Design review of the part shown in the three views and the two pictorial views. Dimensions are in mm from the part's minimum x, y and z. A direction names the side the tool comes from. Give positions to 0.01 mm unless a question says otherwise; leave off trailing zeros. Order: outer loops, then holes, each group sorted by start corner. A loop starts at its lowest first (then second) coordinate and runs counter-clockwise, first axis right, second up.
Item 1: Consider section B-B (y = 12). Give the boundary of the cut face in (x, z), plus the area to 3 significant figures.
Item 2: The part is to be moulded in two halves that separate along X. For the marked faces 1, 2 and 3, say which applies: released by +X, released by -X, zero draft, split by the parting line, or undercut.
Item 3: For probe 1 along Y at (x, z) = (12, 4.4); probe 2 along Z at (x, y) = (12, 14.5); probe 3 along X at (y, z) = (12.25, 9), list the stretches that pass through material, from the lowest coordinate up.
Item 4: Consider section A-A (x = 12). Give the boundary of the cut face in (y, z), plus the area to 3 significant figures.
Item 5: Consider section C-C (z = 7). Give the boundary of the cut face in (x, y).
Item 6: For P1, Ø1.5, axis at x = 5.5, y = 15, coming from the -Z side (1 decimal); P2, Ø8, axis at x = 15.5, y = 6, coming from the -Z side; P3, Ø1, axis at x = 5, z = 10.5, coming from the +Y side; P4, Ø2, axis at x = 3.5, y = 17, coming from the +Z side, all flat-tipped, find the tip position at first contact; note any pin that passes through.
Item 7: Consider section D-D (x = 18.75). Give the boundary of the cut face in (y, z).
Item 8: Machinability: for the marked faces 4 and 5, which of the approach directions +Z, -Z, +X, -X, +Y, -Y give a long, thin tool a straight path to every point of the face, cutting with its end or side? Answer none if there is none.
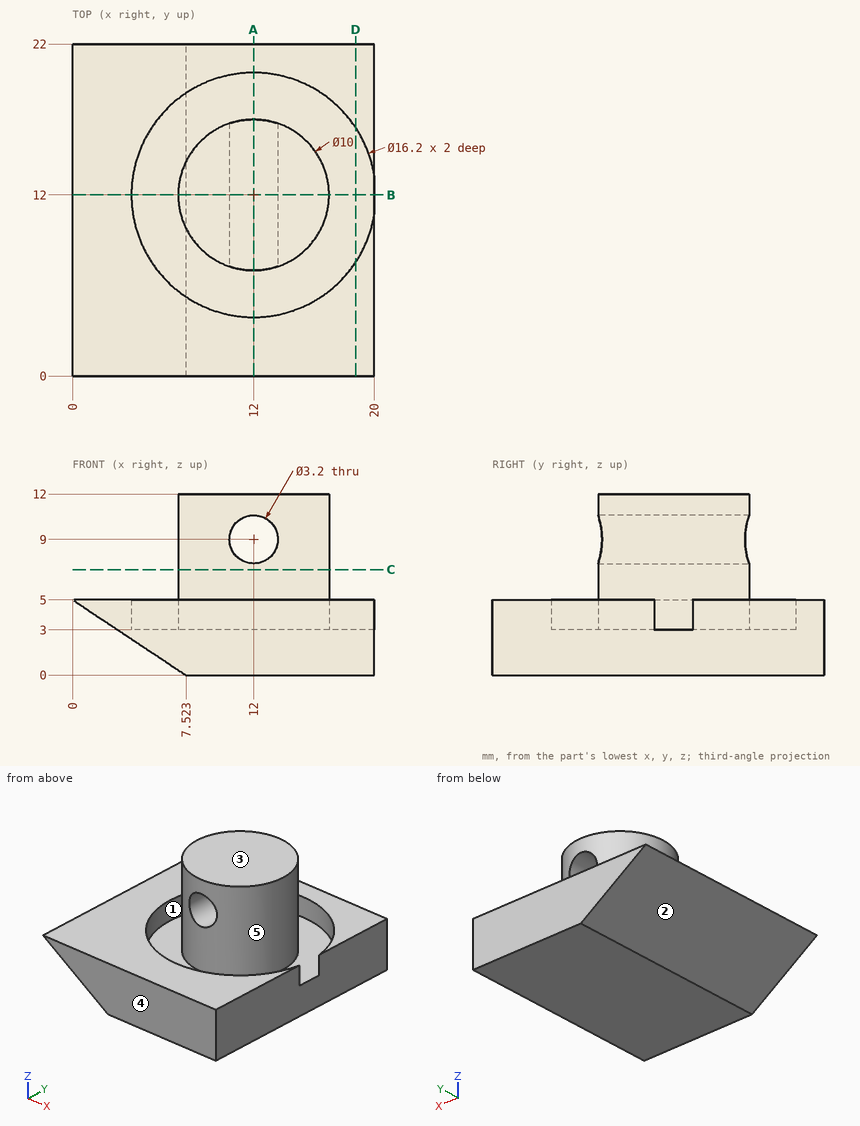
Resolved:
1. outline: (0, 5) - (7.52, 0) - (20, 0) - (20, 3) - (17, 3) - (17, 12) - (7, 12) - (7, 3) - (3.9, 3) - (3.9, 5) - close; hole circle Ø3.2 at (12, 9)
1. area: 131 mm2
2. face 1: undercut
2. face 2: released by -X
2. face 3: zero draft
3. probe 1: y = 0 to 3.9, 7 to 17, 20.1 to 22
3. probe 2: z = 0 to 7.4, 10.6 to 12
3. probe 3: x = 7.01 to 10.4, 13.6 to 16.99
4. outline: (0, 0) - (22, 0) - (22, 5) - (20.1, 5) - (20.1, 3) - (17, 3) - (17, 7.4) - (7, 7.4) - (7, 3) - (3.9, 3) - (3.9, 5) - (0, 5) - close; (7, 10.6) - (17, 10.6) - (17, 12) - (7, 12) - close
4. area: 136 mm2
5. outline: circle Ø10 at (12, 12)
6. P1: stops at z = 0.8
6. P2: stops at z = 0
6. P3: passes through
6. P4: stops at z = 5
7. outline: (0, 0) - (22, 0) - (22, 5) - (16.48, 5) - (16.48, 3) - (7.52, 3) - (7.52, 5) - (0, 5) - close
8. face 4: +Z, -Z, +X, -X, -Y
8. face 5: +Z
